from build123d import *

# Parameters (mm, degrees)
SCHIZZO1_W                   = 35
SCHIZZO1_H                   = 27
ESTRUSIONE_ESTRUSIONE1_DEPTH = 36
SCHIZZO3_R                   = 5
TAGLIO_ESTRUSIONE1_DEPTH     = 28
SCHIZZO4_R                   = 11
TAGLIO_ESTRUSIONE2_DEPTH     = 3.5
SCHIZZO7_W                   = 35
SCHIZZO7_H                   = 36
ESTRUSIONE_ESTRUSIONE3_DEPTH = 5


with BuildPart() as part:
    # Schizzo1 → Estrusione-Estrusione1 (new body)
    with BuildSketch(Plane.XY):
        Rectangle(SCHIZZO1_W, SCHIZZO1_H)
    extrude(amount=ESTRUSIONE_ESTRUSIONE1_DEPTH)

    # Schizzo3 → Taglio-Estrusione1 (cut, through all)
    with BuildSketch(Plane(origin=(0, 13.5, 0), x_dir=(1, 0, 0), z_dir=(0, 1, 0))):
        with Locations((0, -18)):
            Circle(SCHIZZO3_R)
    extrude(amount=-TAGLIO_ESTRUSIONE1_DEPTH, mode=Mode.SUBTRACT)

    # Schizzo4 → Taglio-Estrusione2 (cut)
    with BuildSketch(Plane.XZ.offset(13.5)):
        with Locations((0, 18)):
            Circle(SCHIZZO4_R)
    extrude(amount=-TAGLIO_ESTRUSIONE2_DEPTH, mode=Mode.SUBTRACT)

    # Schizzo7 → Estrusione-Estrusione3 (add)
    with BuildSketch(Plane(origin=(0, 13.5, 0), x_dir=(1, 0, 0), z_dir=(0, 1, 0))):
        with Locations((0, -18)):
            Rectangle(SCHIZZO7_W, SCHIZZO7_H)
    extrude(amount=ESTRUSIONE_ESTRUSIONE3_DEPTH)


solid = part.part
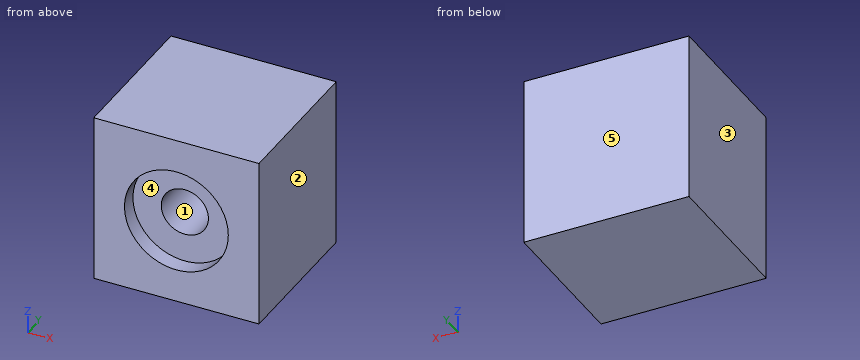
Geometry: final body of the model. Coordinates: model frame, mm. Face numbers are marked on the shaded views. A direction names the side the tool comes from. Give positions to 0.01 mm unless a question says otherwise; leave off trailing zeros. Write each loop counter-clockwise with the first axis right and the second up, starting at its lowest first coordinate (ties: lowest second). Pieces come first, ordered by that corner, then holes. Notation, with made-up numbers: (-2, 37) -> (52, 37) arc R24 cw to (52, 51) -> close; hole circle Ø10 at (40.25, 2.25). An arc over 180 degrees is marked (long way). Answer in a Markdown table with one row per item.
(1) Set-up query: the marked faces 1 and 2. Return all of +Z, -Z, +X, -X, +Y, -Y with unobstructed straight access to the full face (end or side cutting, diameter ignored); none if empty.
Answers below:
| item | result |
|---|---|
| face 1 | -Y |
| face 2 | +Z, -Z, +X, +Y, -Y |
(2) Section query C-C on x = 4.5. Return loops of the section in (y, z).
Answers below:
| item | result |
|---|---|
| outline | (-13.5, 0) -> (18.5, 0) -> (18.5, 36) -> (-13.5, 36) -> (-13.5, 28.04) -> (-10, 28.04) -> (-10, 20.18) -> (13.5, 20.18) -> (13.5, 15.82) -> (-10, 15.82) -> (-10, 7.96) -> (-13.5, 7.96) -> close |
(3) Section query A-A on z = 18. Return loops of the section in (x, y).
Answers below:
| item | result |
|---|---|
| outline | (-17.5, -13.5) -> (-11, -13.5) -> (-11, -10) -> (-5, -10) -> (-5, 13.5) -> (5, 13.5) -> (5, -10) -> (11, -10) -> (11, -13.5) -> (17.5, -13.5) -> (17.5, 18.5) -> (-17.5, 18.5) -> close |
(4) Draft query along X for the marked faces 3, 4 and 5. Return one class per face: +X half, -X half, draft (parallel to the pull), parting line (faces both ways), or undercut.
Answers below:
| item | result |
|---|---|
| face 3 | -X half |
| face 4 | undercut |
| face 5 | draft |
(5) Section query B-B on y = 1. Return loops of the section in (x, z).
Answers below:
| item | result |
|---|---|
| outline | (-17.5, 0) -> (17.5, 0) -> (17.5, 36) -> (-17.5, 36) -> close; hole circle Ø10 at (0, 18) |
(6) Pin query (flat end, axial travel): pin 1 (5 mm diameter, centred on x = -0.5, z = 15.5, fed in from -Y). Return the tip coordinate at first contact, or that it passes through.
Answers below:
| item | result |
|---|---|
| pin 1 | y = -10 |
(7) Ray query, line 1 along X through (y, z) = (-2, 18); line 2 along Z through (x, y) = (0, -11); line 3 along Z through (x, y) = (0, 6.25). Return the intervals inside material, ascending. Write a range as [from, to].
Answers below:
| item | result |
|---|---|
| line 1 | [-17.5, -5], [5, 17.5] |
| line 2 | [0, 7], [29, 36] |
| line 3 | [0, 13], [23, 36] |
(8) Section query D-D on z = 8. Return loops of the section in (x, y).
Answers below:
| item | result |
|---|---|
| outline | (-17.5, -13.5) -> (-4.58, -13.5) -> (-4.58, -10) -> (4.58, -10) -> (4.58, -13.5) -> (17.5, -13.5) -> (17.5, 18.5) -> (-17.5, 18.5) -> close |
